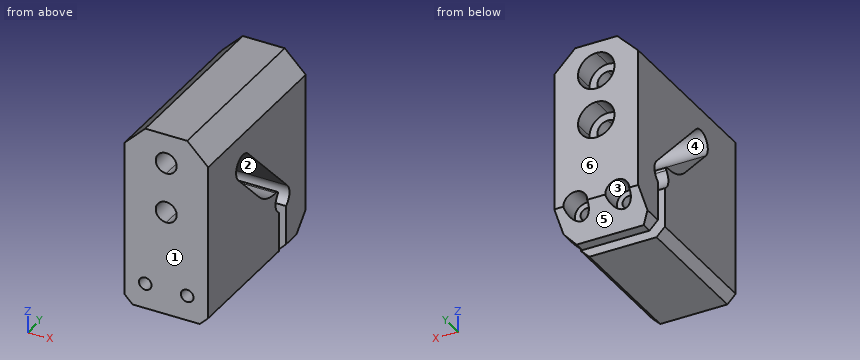
from build123d import *

# Parameters (mm, degrees)
EXTRUDE_1_DEPTH     = 20
FILLET_1_R          = 10
FILLET_2_R          = 0.5
CUT_EXTRUDE_1_DEPTH = 5
CUT_EXTRUDE_2_DEPTH = 5
CUT_EXTRUDE_3_DEPTH = 56.353410012
CHAMFER_1_SIZE      = 5
CHAMFER_2_SIZE      = 2


with BuildPart() as part:
    # Sketch 1 → Extrude 1 (new body)
    with BuildSketch(Plane(origin=(0, 0, 0), x_dir=(0, 0, -1), z_dir=(1, 0, 0))):
        with BuildLine():
            ThreePointArc((-14.849242405, -19.091883092), (-19.091883092, -19.091883092), (-19.091883092, -14.849242405))
            Line((-19.091883092, -14.849242405), (-2.121320344, 2.121320344))
            ThreePointArc((-2.121320344, 2.121320344), (0.391578577, 2.974334584), (2.598076211, 1.5))
            Line((2.598076211, 1.5), (14, 1.5))
            Line((14, 1.5), (14, 4))
            Line((14, 4), (8, 10))
            Line((8, 10), (-30, 10))
            Line((-30, 10), (-30, -32))
            Line((-30, -32), (14, -32))
            Line((14, -32), (14, -1.5))
            Line((14, -1.5), (2.598076211, -1.5))
            ThreePointArc((2.598076211, -1.5), (2.380060021, -1.826284287), (2.121320344, -2.121320344))
            Line((2.121320344, -2.121320344), (-2.903502563, -7.14614325))
            Line((-2.903502563, -7.14614325), (-14.849242405, -19.091883092))
        make_face()
        with BuildLine():
            Line((-2.998906144, -0.081005802), (-2.903502563, -7.14614325))
            Line((-2.903502563, -7.14614325), (2.121320344, -2.121320344))
            ThreePointArc((2.121320344, -2.121320344), (-1.110522429, -2.78688714), (-2.998906144, -0.081005802))
        make_face()
    extrude(amount=EXTRUDE_1_DEPTH)

    # Fillet 1
    fillet_1_edges = [part.edges().sort_by_distance(p)[0] for p in [
        (10, -7.14614325, 2.903502563),
    ]]
    fillet(fillet_1_edges, radius=FILLET_1_R)

    # Fillet 2
    fillet_2_edges = [part.edges().sort_by_distance(p)[0] for p in [
        (10, -0.081005802, 2.998906144),
    ]]
    fillet(fillet_2_edges, radius=FILLET_2_R)

    # Sketch 2 → Cut-Extrude 1 (cut)
    with BuildSketch(Plane(origin=(0, 10, 0), x_dir=(1, 0, 0), z_dir=(0, 1, 0))):
        with BuildLine():
            ThreePointArc((14.35, -11), (13.075914498, -7.924085502), (10, -6.65))
            Line((10, -6.65), (10, -8.5))
            ThreePointArc((10, -8.5), (11.767766953, -9.232233047), (12.5, -11))
            ThreePointArc((12.5, -11), (11.767766953, -12.767766953), (10, -13.5))
            Line((10, -13.5), (10, -15.35))
            ThreePointArc((10, -15.35), (13.075914498, -14.075914498), (14.35, -11))
        make_face()
        with BuildLine():
            Line((10, -8.5), (10, -6.65))
            ThreePointArc((10, -6.65), (5.65, -11), (10, -15.35))
            Line((10, -15.35), (10, -13.5))
            ThreePointArc((10, -13.5), (7.5, -11), (10, -8.5))
        make_face()
        with BuildLine():
            ThreePointArc((14.35, -23), (13.075914498, -19.924085502), (10, -18.65))
            Line((10, -18.65), (10, -20.5))
            ThreePointArc((10, -20.5), (11.767766953, -21.232233047), (12.5, -23))
            ThreePointArc((12.5, -23), (11.767766953, -24.767766953), (10, -25.5))
            Line((10, -25.5), (10, -27.35))
            ThreePointArc((10, -27.35), (13.075914498, -26.075914498), (14.35, -23))
        make_face()
        with BuildLine():
            Line((10, -20.5), (10, -18.65))
            ThreePointArc((10, -18.65), (5.65, -23), (10, -27.35))
            Line((10, -27.35), (10, -25.5))
            ThreePointArc((10, -25.5), (7.5, -23), (10, -20.5))
        make_face()
    extrude(amount=-CUT_EXTRUDE_1_DEPTH, mode=Mode.SUBTRACT)

    # Sketch 2_3 → Cut-Extrude 2 (cut)
    with BuildSketch(Plane(origin=(0, 10, 0), x_dir=(1, 0, 0), z_dir=(0, 1, 0))):
        with BuildLine():
            ThreePointArc((17.85, 8), (15, 10.85), (12.15, 8))
            Line((12.15, 8), (13.5, 8))
            ThreePointArc((13.5, 8), (15, 9.5), (16.5, 8))
            Line((16.5, 8), (17.85, 8))
        make_face()
        with BuildLine():
            Line((13.5, 8), (12.15, 8))
            ThreePointArc((12.15, 8), (15, 5.15), (17.85, 8))
            Line((17.85, 8), (16.5, 8))
            ThreePointArc((16.5, 8), (15, 6.5), (13.5, 8))
        make_face()
        with BuildLine():
            Line((7.85, 8), (6.5, 8))
            ThreePointArc((6.5, 8), (5, 6.5), (3.5, 8))
            Line((3.5, 8), (2.15, 8))
            ThreePointArc((2.15, 8), (5, 5.15), (7.85, 8))
        make_face()
        with BuildLine():
            ThreePointArc((3.5, 8), (5, 9.5), (6.5, 8))
            Line((6.5, 8), (7.85, 8))
            ThreePointArc((7.85, 8), (5, 10.85), (2.15, 8))
            Line((2.15, 8), (3.5, 8))
        make_face()
    extrude(amount=-CUT_EXTRUDE_2_DEPTH, mode=Mode.SUBTRACT)

    # Sketch 2_4 → Cut-Extrude 3 (cut, through all)
    with BuildSketch(Plane(origin=(0, 10, 0), x_dir=(1, 0, 0), z_dir=(0, 1, 0))):
        with BuildLine():
            Line((16.5, 8), (13.5, 8))
            ThreePointArc((13.5, 8), (15, 6.5), (16.5, 8))
        make_face()
        with BuildLine():
            ThreePointArc((16.5, 8), (15, 9.5), (13.5, 8))
            Line((13.5, 8), (16.5, 8))
        make_face()
        with BuildLine():
            Line((3.5, 8), (6.5, 8))
            ThreePointArc((6.5, 8), (5, 9.5), (3.5, 8))
        make_face()
        with BuildLine():
            ThreePointArc((3.5, 8), (5, 6.5), (6.5, 8))
            Line((6.5, 8), (3.5, 8))
        make_face()
        with BuildLine():
            ThreePointArc((12.5, -11), (11.767766953, -9.232233047), (10, -8.5))
            Line((10, -8.5), (10, -13.5))
            ThreePointArc((10, -13.5), (11.767766953, -12.767766953), (12.5, -11))
        make_face()
        with BuildLine():
            Line((10, -13.5), (10, -8.5))
            ThreePointArc((10, -8.5), (7.5, -11), (10, -13.5))
        make_face()
        with BuildLine():
            ThreePointArc((12.5, -23), (11.767766953, -21.232233047), (10, -20.5))
            Line((10, -20.5), (10, -25.5))
            ThreePointArc((10, -25.5), (11.767766953, -24.767766953), (12.5, -23))
        make_face()
        with BuildLine():
            Line((10, -25.5), (10, -20.5))
            ThreePointArc((10, -20.5), (7.5, -23), (10, -25.5))
        make_face()
    extrude(amount=-CUT_EXTRUDE_3_DEPTH, mode=Mode.SUBTRACT)

    # Chamfer 1
    chamfer_1_edges = [part.edges().sort_by_distance(p)[0] for p in [
        (0, -11, 30),
        (20, -11, 30),
    ]]
    chamfer(chamfer_1_edges, length=CHAMFER_1_SIZE)

    # Chamfer 2
    chamfer_2_edges = [part.edges().sort_by_distance(p)[0] for p in [
        (0, -16.75, -14),
        (0, 2.75, -14),
        (20, 2.75, -14),
        (20, -16.75, -14),
    ]]
    chamfer(chamfer_2_edges, length=CHAMFER_2_SIZE)


solid = part.part
Part model, mm, in its own coordinate system. Face numbers are marked on the shaded views. A direction names the side the tool comes from. Give positions to 0.01 mm unless a question says otherwise; leave off trailing zeros. Write each loop counter-clockwise with the first axis right and the second up, starting at its lowest first coordinate (ties: lowest second). Pieces come first, ordered by that corner, then holes.
1) Which spindle directions (+Z, -Z, +X, -X, +Y, -Y) get a long thin tool onto all of the face, cutting with end or side? Do the marked faces 1, 2 and 3. Say none if no direction does.
Resolved:
face 1: +Z, -Z, +X, -X, -Y
face 2: +X, -X
face 3: +Y
2) Cut at D-D on x = 9. State how many separate pieces and enclosed holes the cut face has, then the cut area to 3 significant figures.
Resolved:
separate pieces: 4
enclosed holes: 0
area: 1,250 mm2
3) Cut at B-B on y = -27.5. Write the cut outline in (x, z).
Resolved:
outline: (0, -12) - (2, -14) - (18, -14) - (20, -12) - (20, 25) - (15, 30) - (5, 30) - (0, 25) - close; hole circle Ø3 at (5, -8); hole circle Ø5 at (10, 11); hole circle Ø5 at (10, 23); hole circle Ø3 at (15, -8)
4) Probe L1, parallel to X at y = 4, z = -8; L2, parallel to Y at x = 10, z = -5; L3, parallel to Y at x = 4.25, z = -5.5. List the from-to ranges inside material, lowest first.
Resolved:
L1: x = 0 to 3.5, 6.5 to 13.5, 16.5 to 20
L2: y = -32 to -1.5, 1.5 to 10
L3: y = -32 to -1.5, 1.5 to 5
5) Cut at A-A on y = -14. Write the cut outline in (x, z), then the cut area to 3 significant figures.
Resolved:
outline: (0, -12) - (2, -14) - (18, -14) - (20, -12) - (20, 9.76) - (12.17, 9.76) arc R2.5 cw to (7.83, 9.76) - (0, 9.76) - close; (0, 18.24) - (20, 18.24) - (20, 25) - (15, 30) - (5, 30) - (0, 25) - close; hole circle Ø3 at (5, -8); hole circle Ø5 at (10, 23); hole circle Ø3 at (15, -8)
area: 644 mm2
6) Two-plate mould, pull along Z, no slides. Class the marked faces 4, 5 and 6: released by +Z, released by -Z, zero draft, split by the parting line, or undercut.
Resolved:
face 4: undercut
face 5: released by -Z
face 6: zero draft
7) Pin check, flat tip, straight feed: pin 1 (4 mm diameter, centred on x = 15, z = -8, fed in from +Y). Stop position of the tip, or through.
Resolved:
pin 1: stops at y = 5
8) Cut at C-C on z = 18. Write the cut outline in (x, y).
Resolved:
outline: (0, -32) - (20, -32) - (20, -19.79) - (0, -19.79) - close; (0, -13.76) - (20, -13.76) - (20, 10) - (0, 10) - close
